```python
from build123d import *

# Parameters (mm, degrees)
ESQUISSE1_W             = 96.6
ESQUISSE1_H             = 32
BOSS_EXTRU_1_DEPTH      = 2.2
ESQUISSE6_R             = 3.45
BOSS_EXTRU_2_DEPTH      = 32.6
ESQUISSE7_R             = 3
ENL_V_MAT_EXTRU_1_DEPTH = 35.8


with BuildPart() as part:
    # Esquisse1 → Boss.-Extru.1 (new body)
    with BuildSketch(Plane.XY):
        with Locations((0.671156739, 2.259938231)):
            Rectangle(ESQUISSE1_W, ESQUISSE1_H)
    extrude(amount=BOSS_EXTRU_1_DEPTH)

    # Esquisse6 → Boss.-Extru.2 (add)
    with BuildSketch(Plane.XY.offset(2.2)):
        with Locations((-31.628843261, 2.259938231)):
            Circle(ESQUISSE6_R)
        with Locations((32.971156739, 2.259938231)):
            Circle(ESQUISSE6_R)
    extrude(amount=BOSS_EXTRU_2_DEPTH)

    # Esquisse7 → Enlèv. mat.-Extru.1 (cut, through all)
    with BuildSketch(Plane.XY.offset(34.8)):
        with Locations((-31.628843261, 2.259938231)):
            Circle(ESQUISSE7_R)
        with Locations((32.971156739, 2.259938231)):
            Circle(ESQUISSE7_R)
        with BuildLine():
            Line((-14.328843261, 7.259938231), (15.671156739, 7.259938231))
            ThreePointArc((15.671156739, 7.259938231), (20.671156739, 2.259938231), (15.671156739, -2.740061769))
            Line((15.671156739, -2.740061769), (-14.328843261, -2.740061769))
            ThreePointArc((-14.328843261, -2.740061769), (-19.328843261, 2.259938231), (-14.328843261, 7.259938231))
        make_face()
    extrude(amount=-ENL_V_MAT_EXTRU_1_DEPTH, mode=Mode.SUBTRACT)


solid = part.part
```
Work out the finished part from the listing and answer in its coordinate system (mm). A direction names the side the tool comes from. Coordinates: 2 decimals unless noted, no trailing zeros. Loops run counter-clockwise (first coordinate to the right, second up) from the corner with the lowest first, then second, coordinate; pieces in that order, holes last.
1) Section B-B (y = 1) is taken. Give the vertices of the cut face in (x, z).
Results:
outline: (-47.63, 0) - (-34.35, 0) - (-34.35, 34.8) - (-34.84, 34.8) - (-34.84, 2.2) - (-47.63, 2.2) - close; (-28.91, 0) - (-19.17, 0) - (-19.17, 2.2) - (-28.42, 2.2) - (-28.42, 34.8) - (-28.91, 34.8) - close; (20.51, 0) - (30.25, 0) - (30.25, 34.8) - (29.76, 34.8) - (29.76, 2.2) - (20.51, 2.2) - close; (35.69, 0) - (48.97, 0) - (48.97, 2.2) - (36.18, 2.2) - (36.18, 34.8) - (35.69, 34.8) - close
2) For faces 1 (the flat face through (1, -2.74, 1)), 2 (the cylindrical face through (29.524, 2.412, 18.272)), 3 (the flat face through (0, 18.26, 1)), determine the directions among +Z, -Z, +X, -X, +Y, -Y from which every point of the face is accessible in a straight line to the end or side of a thin tool.
Results:
face 1: +Z, -Z
face 2: +Z
face 3: +Z, -Z, +X, -X, +Y
3) Consider probe 1 along Y at (x, z) = (33, 19.5); probe 2 along X at (y, z) = (5, 28.5); probe 3 along X at (y, z) = (2, 21). Determine where each line is inside the solid, lowest interval first.
Results:
probe 1: y = -1.19 to -0.74, 5.26 to 5.71
probe 2: x = -33.73 to -32.85, -30.41 to -29.53, 30.87 to 31.75, 34.19 to 35.07
probe 3: x = -35.07 to -34.62, -28.64 to -28.19, 29.53 to 29.98, 35.96 to 36.41
4) For a pull along Y with two mould halves and no side action, classify faces 4 (the flat face through (48.971, 2, 1)), 5 (the cylindrical face through (-35.076, 2.412, 18.272)), 6 (the cylindrical face through (-19.328, 2.15, 1.115)) as +Y half, -Y half, draft (parallel to the pull), parting line (faces both ways), or undercut.
Results:
face 4: draft
face 5: parting line
face 6: undercut
5) Section D-D (y = 13) is taken. Give the vertices of the cut face in (x, z), plus the area to 3 significant figures.
Results:
outline: (-47.63, 0) - (48.97, 0) - (48.97, 2.2) - (-47.63, 2.2) - close
area: 213 mm2
6) Section A-A (x = -10.5) is taken. Give the vertices of the cut face in (y, z), plus the area to 3 significant figures.
Results:
outline: (-13.74, 0) - (-2.74, 0) - (-2.74, 2.2) - (-13.74, 2.2) - close; (7.26, 0) - (18.26, 0) - (18.26, 2.2) - (7.26, 2.2) - close
area: 48.4 mm2
7) Section C-C (z = 17) is taken. Give the vertices of the cut face in (x, y).
Results:
outline: circle Ø6.9 at (-31.63, 2.26); circle Ø6.9 at (32.97, 2.26); hole circle Ø6 at (-31.63, 2.26); hole circle Ø6 at (32.97, 2.26)
8) Flat-ended cylindrical pins translate along their axes: pin 1 (5 mm diameter, centred on y = 7, z = 11, fed in from +X) (3 decimals); pin 2 (6 mm diameter, centred on y = 5, z = 11.5, fed in from -X); pin 3 (8 mm diameter, centred on x = -25, z = 17.5, fed in from +Y); pin 4 (12 mm diameter, centred on x = 16.5, z = 11.5, fed in from +Y). Find the tip coordinate at first contact, or state that the pin passes through.
Results:
pin 1: stops at x = 35.595
pin 2: stops at x = -35.08
pin 3: stops at y = 4.49
pin 4: passes through
